```python
from build123d import *

# Parameters (mm, degrees)
SKETCH1_W               = 313.367
SKETCH1_H               = 315.36
SKETCH1_W_2             = 309.367
SKETCH1_H_2             = 311.36
EXTRUDE_THIN1_DEPTH     = 119
CUT_EXTRUDE1_DEPTH      = 445.128605574
CUT_EXTRUDE1_DEPTH_BACK = 445.128605574
SKETCH3_W               = 2
SKETCH3_H               = 12
BOSS_EXTRUDE1_DEPTH     = 12
SKETCH4_W               = 2
SKETCH4_H               = 12
BOSS_EXTRUDE2_DEPTH     = 12
SKETCH5_W               = 2
SKETCH5_H               = 12
BOSS_EXTRUDE3_DEPTH     = 12
SKETCH6_W               = 2
SKETCH6_H               = 12
BOSS_EXTRUDE4_DEPTH     = 12
CUT_EXTRUDE2_DEPTH      = 392.361567721


with BuildPart() as part:
    # Sketch1 → Extrude-Thin1 (new body)
    with BuildSketch(Plane.XY):
        with Locations((134.6835, -44.32)):
            Rectangle(SKETCH1_W, SKETCH1_H)
        with Locations((134.6835, -44.32)):
            Rectangle(SKETCH1_W_2, SKETCH1_H_2, mode=Mode.SUBTRACT)
    extrude(amount=EXTRUDE_THIN1_DEPTH)

    # Sketch2 → Cut-Extrude1 (cut, two sides: drawn at the far end of the back side and taken through both)
    with BuildSketch(Plane(origin=(0, -200, 0), x_dir=(1, 0, 0), z_dir=(0, 1, 0)).offset(-CUT_EXTRUDE1_DEPTH_BACK)):
        with BuildLine():
            Line((39, -13), (81.6835, -13))
            ThreePointArc((81.6835, -13), (128.6835, -60), (81.6835, -107))
            Line((81.6835, -107), (39, -107))
            ThreePointArc((39, -107), (-8, -60), (39, -13))
        make_face()
        with BuildLine():
            Line((187.6835, -13), (230.367, -13))
            ThreePointArc((230.367, -13), (277.367, -60), (230.367, -107))
            Line((230.367, -107), (187.6835, -107))
            ThreePointArc((187.6835, -107), (140.6835, -60), (187.6835, -13))
        make_face()
    extrude(amount=CUT_EXTRUDE1_DEPTH + CUT_EXTRUDE1_DEPTH_BACK, mode=Mode.SUBTRACT)

    # Sketch3 → Boss-Extrude1 (add)
    with BuildSketch(Plane(origin=(-20, 0, 0), x_dir=(0, 0, -1), z_dir=(1, 0, 0))):
        with Locations((-2, -194)):
            Rectangle(SKETCH3_W, SKETCH3_H)
    extrude(amount=BOSS_EXTRUDE1_DEPTH)

    # Sketch4 → Boss-Extrude2 (add)
    with BuildSketch(Plane(origin=(-20, 0, 0), x_dir=(0, 0, -1), z_dir=(1, 0, 0))):
        with Locations((-2, 105.36)):
            Rectangle(SKETCH4_W, SKETCH4_H)
    extrude(amount=BOSS_EXTRUDE2_DEPTH)

    # Sketch5 → Boss-Extrude3 (add)
    with BuildSketch(Plane.ZY.offset(-289.367)):
        with Locations((2, 105.36)):
            Rectangle(SKETCH5_W, SKETCH5_H)
    extrude(amount=BOSS_EXTRUDE3_DEPTH)

    # Sketch6 → Boss-Extrude4 (add)
    with BuildSketch(Plane.ZY.offset(-289.367)):
        with Locations((2, -194)):
            Rectangle(SKETCH6_W, SKETCH6_H)
    extrude(amount=BOSS_EXTRUDE4_DEPTH)

    # Sketch7 → Cut-Extrude2 (cut, through all)
    with BuildSketch(Plane(origin=(291.367, 0, 0), x_dir=(0, 0, -1), z_dir=(1, 0, 0))):
        with BuildLine():
            Line((-91, 101.36), (-28, 101.36))
            ThreePointArc((-28, 101.36), (-9.331428571, 82.691428571), (-28, 64.022857143))
            Line((-28, 64.022857143), (-91, 64.022857143))
            ThreePointArc((-91, 64.022857143), (-109.668571429, 82.691428571), (-91, 101.36))
        make_face()
        with BuildLine():
            Line((-91, 59.022857143), (-28, 59.022857143))
            ThreePointArc((-28, 59.022857143), (-9.331428571, 40.354285714), (-28, 21.685714286))
            Line((-28, 21.685714286), (-91, 21.685714286))
            ThreePointArc((-91, 21.685714286), (-109.668571429, 40.354285714), (-91, 59.022857143))
        make_face()
        with BuildLine():
            Line((-91, 16.685714286), (-28, 16.685714286))
            ThreePointArc((-28, 16.685714286), (-9.331428571, -1.982857143), (-28, -20.651428571))
            Line((-28, -20.651428571), (-91, -20.651428571))
            ThreePointArc((-91, -20.651428571), (-109.668571429, -1.982857143), (-91, 16.685714286))
        make_face()
        with BuildLine():
            Line((-91, -25.651428571), (-28, -25.651428571))
            ThreePointArc((-28, -25.651428571), (-9.331428571, -44.32), (-28, -62.988571429))
            Line((-28, -62.988571429), (-91, -62.988571429))
            ThreePointArc((-91, -62.988571429), (-109.668571429, -44.32), (-91, -25.651428571))
        make_face()
        with BuildLine():
            Line((-91, -67.988571429), (-28, -67.988571429))
            ThreePointArc((-28, -67.988571429), (-9.331428571, -86.657142857), (-28, -105.325714286))
            Line((-28, -105.325714286), (-91, -105.325714286))
            ThreePointArc((-91, -105.325714286), (-109.668571429, -86.657142857), (-91, -67.988571429))
        make_face()
        with BuildLine():
            Line((-91, -110.325714286), (-28, -110.325714286))
            ThreePointArc((-28, -110.325714286), (-9.331428571, -128.994285714), (-28, -147.662857143))
            Line((-28, -147.662857143), (-91, -147.662857143))
            ThreePointArc((-91, -147.662857143), (-109.668571429, -128.994285714), (-91, -110.325714286))
        make_face()
        with BuildLine():
            Line((-91, -152.662857143), (-28, -152.662857143))
            ThreePointArc((-28, -152.662857143), (-9.331428571, -171.331428571), (-28, -190))
            Line((-28, -190), (-91, -190))
            ThreePointArc((-91, -190), (-109.668571429, -171.331428571), (-91, -152.662857143))
        make_face()
    extrude(amount=-CUT_EXTRUDE2_DEPTH, mode=Mode.SUBTRACT)


solid = part.part
```
Part model, mm, in its own coordinate system. A direction names the side the tool comes from. Coordinates: 2 decimals unless noted, no trailing zeros. Write each loop counter-clockwise with the first axis right and the second up, starting at its lowest first coordinate (ties: lowest second). Pieces come first, ordered by that corner, then holes.
Item 1: Slice it at B-B (x = 207.5). Write the cut outline in (y, z), and give its area (3 significant figures).
Item 2: Probe line 1 (Y direction, x = 235, z = 108.5); line 2 (X direction, y = 33, z = 112.5). List the from-to ranges inside material, lowest first.
Item 3: Which spindle directions (+Z, -Z, +X, -X, +Y, -Y) get a long thin tool onto all of the face, cutting with end or side? Do faces 1 (the face through (290.381, -129.405, 109.664)), 2 (the face through (291.367, -22, 64)), 3 (the face through (-14, -194, 3)), 4 (the face through (283, -194, 1)), 5 (the face through (140.695, -201.014, 61.034)). Say none if no direction does.
Item 4: Pin check, flat tip, straight feed: pin 1 (10 mm diameter, centred on x = 177, z = 23.5, fed in from -Y). Stop position of the tip, or through.
Item 5: Mould opens along Y. For faces 6 (the face through (277.356, -201.014, 58.966)), 7 (the face through (283, 105, 3)) say: released by +Y, released by -Y, zero draft, split by the parting line, or undercut.
Item 6: Slice it at C-C (z = 60). Count the separate pieces of the cut face and the enclosed holes in it, and give its area (3 significant figures).
Item 7: Slice it at A-A (y = -44.32). Write the cut outline in (x, z), and give its area (3 significant figures).
Results found:
1. outline: (-202, 0) - (-200, 0) - (-200, 13) - (-202, 13) - close; (-202, 107) - (-200, 107) - (-200, 119) - (-202, 119) - close; (111.36, 0) - (113.36, 0) - (113.36, 13) - (111.36, 13) - close; (111.36, 107) - (113.36, 107) - (113.36, 119) - (111.36, 119) - close
1. area: 100 mm2
2. line 1: y = -202 to -200, 111.36 to 113.36
2. line 2: x = -22 to -20, 289.37 to 291.37
3. face 1: +X, -X
3. face 2: +Z, -Z, +X, +Y, -Y
3. face 3: +Z
3. face 4: -Z
3. face 5: +Y, -Y
4. pin 1: passes through
5. face 6: zero draft
5. face 7: undercut
6. separate pieces: 18
6. enclosed holes: 0
6. area: 360 mm2
7. outline: (-22, 0) - (-20, 0) - (-20, 9.33) - (-22, 9.33) - close; (-22, 109.67) - (-20, 109.67) - (-20, 119) - (-22, 119) - close; (289.37, 0) - (291.37, 0) - (291.37, 9.33) - (289.37, 9.33) - close; (289.37, 109.67) - (291.37, 109.67) - (291.37, 119) - (289.37, 119) - close
7. area: 74.7 mm2
